Read the model definition and answer for the solid it produces. Units are mm, in the model's axes. A direction names the side the tool comes from. Coordinates: 2 decimals unless noted, no trailing zeros. Loops run counter-clockwise (first coordinate to the right, second up) from the corner with the lowest first, then second, coordinate; pieces in that order, holes last. Notation, with made-up numbers: (15.25, 10.5) -> (24.25, 10.5) arc R12 cw to (24.25, 25.5) -> close; hole circle Ø6 at (85.25, -38.5). An arc over 180 degrees is marked (long way). Answer in a Markdown table with one row per item.
```python
from build123d import *

# Parameters (mm, degrees)
BOSS_EXTRUDE1_DEPTH   = 100
CUT_EXTRUDE1_START    = -28.129025
CUT_EXTRUDE1_DEPTH    = 28.129025
BOSS_EXTRUDE2_DEPTH   = 70
BOSS_EXTRUDE2_2_DEPTH = 70
BOSS_EXTRUDE2_3_DEPTH = 70
BOSS_EXTRUDE2_4_DEPTH = 70
CUT_EXTRUDE2_START    = -20.520945
CUT_EXTRUDE2_DEPTH    = 38.356397
BOSS_EXTRUDE4_DEPTH   = 2


with BuildPart() as part:
    # Sketch2 → Boss-Extrude1 (new body)
    with BuildSketch(Plane(origin=(0, 0, 0), x_dir=(0, 0, -1), z_dir=(1, 0, 0))):
        Polygon((0, 0), (20, 28.562960135), (-20, 28.562960135), align=None)
    extrude(amount=BOSS_EXTRUDE1_DEPTH)

    # Sketch3 → Cut-Extrude1 (cut)
    with BuildSketch(Plane(origin=(0, 28.562960135, 0), x_dir=(1, 0, 0), z_dir=(0, 1, 0)).offset(CUT_EXTRUDE1_START)):
        Polygon((96.527036447, 20), (100, 0.30384494), (100, 20), align=None)
        Polygon((0, 0.30384494), (3.472963553, 20), (0, 20), align=None)
        Polygon((96.527036447, -20), (100, -0.30384494), (100, -20), align=None)
        Polygon((0, -0.30384494), (3.472963553, -20), (0, -20), align=None)
    extrude(amount=CUT_EXTRUDE1_DEPTH, mode=Mode.SUBTRACT)

    # Sketch7 → Cut-Extrude2 (cut)
    with BuildSketch(Plane.XY.offset(CUT_EXTRUDE2_START)):
        Polygon((0, 28.562960135), (28.562960135, 0), (0, 0), align=None)
        Polygon((100, 28.562960135), (100, 0), (71.437039865, 0), align=None)
    extrude(amount=CUT_EXTRUDE2_DEPTH, mode=Mode.SUBTRACT)



with BuildPart() as body_2:
    # Sketch4 → Boss-Extrude2 (new body)
    with BuildSketch(Plane(origin=(0, 28.562960135, 0), x_dir=(1, 0, 0), z_dir=(0, 1, 0))):
        Polygon((3.472963553, 20), (0.518540294, 20.520944533), (-2.954423259, 0.824789473), (0, 0.30384494), align=None)
    extrude(amount=-BOSS_EXTRUDE2_DEPTH)


with BuildPart() as body_3:
    # Sketch4 → Boss-Extrude2 2 (new body)
    with BuildSketch(Plane(origin=(0, 28.562960135, 0), x_dir=(1, 0, 0), z_dir=(0, 1, 0))):
        Polygon((96.527036447, 20), (100, 0.30384494), (102.954423259, 0.824789473), (99.481459706, 20.520944533), align=None)
    extrude(amount=-BOSS_EXTRUDE2_2_DEPTH)


with BuildPart() as body_4:
    # Sketch4 → Boss-Extrude2 3 (new body)
    with BuildSketch(Plane(origin=(0, 28.562960135, 0), x_dir=(1, 0, 0), z_dir=(0, 1, 0))):
        Polygon((96.527036447, -20), (99.481459706, -20.520944533), (102.954423259, -0.824789473), (100, -0.30384494), align=None)
    extrude(amount=-BOSS_EXTRUDE2_3_DEPTH)


with BuildPart() as body_5:
    # Sketch4 → Boss-Extrude2 4 (new body)
    with BuildSketch(Plane(origin=(0, 28.562960135, 0), x_dir=(1, 0, 0), z_dir=(0, 1, 0))):
        Polygon((3.472963553, -20), (0, -0.30384494), (-2.954423259, -0.824789473), (0.518540294, -20.520944533), align=None)
    extrude(amount=-BOSS_EXTRUDE2_4_DEPTH)


with BuildPart() as part_1:
    add(part.part)

    add(body_2.part)  # Boss-Extrude4 merges body 2

    add(body_3.part)  # Boss-Extrude4 merges body 3

    add(body_4.part)  # Boss-Extrude4 merges body 4

    add(body_5.part)  # Boss-Extrude4 merges body 5
    # Sketch8 → Boss-Extrude4 (add)
    with BuildSketch(Plane(origin=(0, 28.562960135, 0), x_dir=(1, 0, 0), z_dir=(0, 1, 0))):
        Polygon((0.518540294, 20.520944533), (26.562031148, 30), (73.437968852, 30), (99.481459706, 20.520944533), (102.954423259, 0.824789473), (102.954423259, -0.824789473), (99.481459706, -20.520944533), (73.437968852, -30), (26.562031148, -30), (0.518540294, -20.520944533), (-2.954423259, -0.824789473), (-2.954423259, 0.824789473), align=None)
    extrude(amount=BOSS_EXTRUDE4_DEPTH)


solid = part_1.part
```
1. Find the intervals of material crossed by probe 1 along X at (y, z) = (10.5, 1.5); probe 2 along X at (y, z) = (7, 1); probe 3 along Y at (x, z) = (29, 27.5), in increasing order.
A:
| item | result |
|---|---|
| probe 1 | x = -2.84 to 0.21, 18.06 to 81.94, 99.79 to 102.84 |
| probe 2 | x = -2.92 to 0.12, 21.56 to 78.44, 99.88 to 102.92 |
| probe 3 | y = 28.56 to 30.56 |
2. The mould has two halves that part along Z. Classify faces 5 (the flat face through (51, 28.563, 24)), 6 (the flat face through (98.24, -5.95, -10.29)), 7 (the flat face through (86.642, 29.549, 25.194)): pulls with the +Z half, pulls with the -Z half, needs draft (parallel to the pull), parting line crosses it, or undercut.
A:
| item | result |
|---|---|
| face 5 | needs draft |
| face 6 | undercut |
| face 7 | pulls with the +Z half |
3. A cutting plane is placed at A-A on y = -17. Give the vertices of the cut face in (x, z), and give its area (3 significant figures).
A:
| item | result |
|---|---|
| outline | (-2.95, -0.82) -> (0.52, -20.52) -> (3.47, -20) -> (0, -0.3) -> close; (-2.95, 0.82) -> (0, 0.3) -> (3.47, 20) -> (0.52, 20.52) -> close; (96.53, -20) -> (99.48, -20.52) -> (102.95, -0.82) -> (100, -0.3) -> close; (96.53, 20) -> (100, 0.3) -> (102.95, 0.82) -> (99.48, 20.52) -> close |
| area | 240 mm2 |
4. A tool of negligible diameter and unlimited length cuts with its end or side. For faces 1 (the flat face through (2.016, -5.947, -20.257)), 2 (the flat face through (101.5, -5.95, 0.57)), 3 (the flat face through (-1.5, -5.95, -0.57)), 4 (the flat face through (88.692, 17.255, -0.25)), from which of +Z, -Z, +X, -X, +Y, -Y can it reach the whole face along a straight path? Write none if from no direction.
A:
| item | result |
|---|---|
| face 1 | -Z, -Y |
| face 2 | +X, -Y |
| face 3 | -X, -Y |
| face 4 | -Y |
5. A cutting plane is placed at D-D on z = -9. Give the vertices of the cut face in (x, y), and give its area (3 significant figures).
A:
| item | result |
|---|---|
| outline | (-1.51, -41.44) -> (1.53, -41.44) -> (1.53, 27.03) -> (15.71, 12.85) -> (84.29, 12.85) -> (98.47, 27.03) -> (98.47, -41.44) -> (101.51, -41.44) -> (101.51, 30.56) -> (-1.51, 30.56) -> close |
| area | 1,950 mm2 |
6. A cutting plane is placed at B-B on y = 18.5. Give the vertices of the cut face in (x, z).
A:
| item | result |
|---|---|
| outline | (-2.95, -0.82) -> (0.52, -20.52) -> (3.47, -20) -> (0, -0.3) -> close; (-2.95, 0.82) -> (0, 0.3) -> (3.47, 20) -> (0.52, 20.52) -> close; (10.06, -12.95) -> (89.94, -12.95) -> (89.94, 12.95) -> (10.06, 12.95) -> close; (96.53, -20) -> (99.48, -20.52) -> (102.95, -0.82) -> (100, -0.3) -> close; (96.53, 20) -> (100, 0.3) -> (102.95, 0.82) -> (99.48, 20.52) -> close |
7. Given pin 1 Ø6 at (y, z) = (-27, 17) entering from -X; pin 2 Ø1.5 at (y, z) = (-31, -16.5) entering from +X; pin 3 Ø12 at (x, z) = (41.5, 4.5) entering from -Y, each flat-ended and moving along its own axis, determine where each tip first touches the part or whether it passes through.
A:
| item | result |
|---|---|
| pin 1 | stops at x = -0.63 |
| pin 2 | stops at x = 100.32 |
| pin 3 | stops at y = 0 |
8. A cutting plane is placed at C-C on x = 43. Give the vertices of the cut face in (y, z).
A:
| item | result |
|---|---|
| outline | (0, 0) -> (28.56, -20) -> (28.56, -30) -> (30.56, -30) -> (30.56, 30) -> (28.56, 30) -> (28.56, 20) -> close |
